from build123d import *

# Parameters (mm, degrees)
BOSS_EXTRUDE1_DEPTH = 3


with BuildPart() as part:
    # Sketch1 → Boss-Extrude1 (new body)
    with BuildSketch(Plane(origin=(0, 0, 0), x_dir=(1, 0, 0), z_dir=(0, 1, 0))):
        with BuildLine():
            Line((0, -130), (0, -105))
            Line((0, -105), (-10, -105))
            Line((-10, -105), (-10, 0))
            Line((-10, 0), (0, 0))
            Line((0, 0), (0, 25))
            Line((0, 25), (219.162, -128.458884489))
            Line((219.162, -128.458884489), (219.162, -187.421055539))
            ThreePointArc((219.162, -187.421055539), (218.770761429, -188.214408879), (217.903180955, -188.386981365))
            Line((217.903180955, -188.386981365), (0, -130))
        make_face()
    extrude(amount=BOSS_EXTRUDE1_DEPTH)


solid = part.part
Build history of the part. All positions in model axes, mm. Coordinates: 2 decimals unless noted, no trailing zeros. Order: outer loops, then holes, each group sorted by start corner. A loop starts at its lowest first (then second) coordinate and runs counter-clockwise, first axis right, second up. Notation, with made-up numbers: (61, 50.5) -> (108, 50.5) arc R10 cw to (108, 58.5) -> close; hole circle Ø3 at (-19.5, 17). An arc over 180 degrees is marked (long way). One line per item, written item: value.
(1) Slice it at A-A, the plane y = 1.4. List the corners of the cut face in (x, z).
Checked values:
outline: (-10, 0) -> (0, 0) -> (0, -25) -> (219.16, 128.46) -> (219.16, 187.42) arc R1 ccw to (217.9, 188.39) -> (0, 130) -> (0, 105) -> (-10, 105) -> close
(2) Probe line 1 (X direction, y = 2.15, z = 48.5); line 2 (Z direction, x = 59.5, y = 1.85); line 3 (X direction, y = 1.4, z = -5). List the from-to ranges inside material, lowest first. Write a range as [from, to].
Checked values:
line 1: [-10, 104.97]
line 2: [16.66, 145.94]
line 3: [0, 28.56]
(3) Drop flat-ended pins along their axis: pin 1 Ø1.5 at (y, z) = (1.5, 120.5) entering from -X; pin 2 Ø1.5 at (y, z) = (2, 60) entering from +X; pin 3 Ø0.9 at (x, y) = (-3.5, 1) entering from -Z. Give the stop position or say it passes through.
Checked values:
pin 1: x = 0
pin 2: x = 122.46
pin 3: z = 0
(4) Slice it at B-B, the plane z = 27. List the corners of the cut face in (x, y), plus the area to 3 significant figures.
Checked values:
outline: (-10, 0) -> (74.26, 0) -> (74.26, 3) -> (-10, 3) -> close
area: 253 mm2
(5) Slice it at C-C, the plane x = 77. List the corners of the cut face in (y, z).
Checked values:
outline: (0, 28.92) -> (3, 28.92) -> (3, 150.63) -> (0, 150.63) -> close
